The model under review builds one solid part; all positions refer to its coordinate system, in mm. A direction names the side the tool comes from. Coordinates: 2 decimals unless noted, no trailing zeros. Write each loop counter-clockwise with the first axis right and the second up, starting at its lowest first coordinate (ties: lowest second). Pieces come first, ordered by that corner, then holes. Notation, with made-up numbers: M 67,-27.5 L 102,-27.5 A32 cw 102,1.5 Z; hole C -4.75,-16.75 d5. An arc over 180 degrees is marked long. Answer as a JSON object with one key per item and string values.
Autodesk Inventor part; units mm, degrees
ref_plane "YZ Plane" through (0, 0, 0) normal (1, 0, 0) x (0, 1, 0)
ref_plane "XZ Plane" through (0, 0, 0) normal (0, 1, 0) x (-1, 0, 0)
ref_plane "XY Plane" through (0, 0, 0) normal (0, 0, 1) x (1, 0, 0)
sketch "Sketch1" plane through (0, 0, 0) normal (0, 0, 1) x (1, 0, 0)
  line L0 (0, 0) -> (12.7, 0)
  line L1 (12.7, 0) -> (12.7, 25.4)
  line L2 (12.7, 25.4) -> (0, 25.4)
  line L3 (0, 25.4) -> (0, 0)
  line L4 (1.27, 24.13) -> (11.43, 24.13)
  line L5 (11.43, 24.13) -> (11.43, 1.27)
  line L6 (11.43, 1.27) -> (1.27, 1.27)
  line L7 (1.27, 1.27) -> (1.27, 24.13)
  dimension "d0" = 25.4
  dimension "d1" = 12.7
  dimension "d2" = 1.27
extrude "Extrusion1" add sketch "Sketch1" along normal blind 203.2
sketch "Sketch2" plane through (12.7, 0, 0) normal (1, 0, 0) x (0, 0, -1)
  line L0 (-168.1044, 12.7) -> (-15.152, 12.7) construction
  line L1 (0, 0) -> (-203.2, 0) construction
  line L2 (-203.2, 0) -> (-203.2, 25.4)
  line L3 (0, 0) -> (0, 25.4)
  point P0 (-177.8, 12.7)
  point P1 (-25.4, 12.7)
  dimension "d5" = 12.7
  dimension "d6" = 25.4
  dimension "d7" = 25.4
hole "Hole1" at (12.7, 12.7, 177.8) at (12.7, 12.7, 25.4) direction (-1, 0, 0) diameter 3.2639 end through all
sketch "Sketch3" plane through (12.7, 0, 0) normal (1, 0, 0) x (0, 0, -1)
  circle A0 centre (-177.8, 12.7) radius 1.632
  circle A1 centre (-25.4, 12.7) radius 1.632
  line L0 (-214.4228, 12.7) -> (16.7128, 12.7) construction
  point P0 (0, 0)
  point P1 (-139.7, 12.7)
  point P2 (-63.5, 12.7)
  dimension "d18" = 38.1
  dimension "d19" = 38.1
hole "Hole2" at (12.7, 12.7, 139.7) at (12.7, 12.7, 63.5) direction (-1, 0, 0) diameter 6.5278 end through all
sketch "Sketch4" plane through (0, 25.4, 0) normal (0, 1, 0) x (1, 0, 0)
  line L0 (6.35, 23.2485) -> (6.35, -226.9955) construction
  line L1 (12.7, 0) -> (12.7, -203.2) construction
  line L2 (12.7, 0) -> (0, 0)
  line L3 (0, 0) -> (0, -203.2)
  line L4 (12.7, -203.2) -> (0, -203.2)
  line L5 (12.7, 0) -> (12.7, -203.2)
  point P0 (0, 0)
  point P1 (6.35, -31.75)
  point P2 (6.35, -171.45)
  dimension "d27" = 6.35
  dimension "d28" = 31.75
  dimension "d29" = 31.75
hole "Hole3" at (6.35, 25.4, 31.75) at (6.35, 25.4, 171.45) direction (0, -1, 0) diameter 3.2512 end through all
properties part number "000101"
(1) For faces 1 (the face through (6, 24.13, 100)), 2 (the face through (12.06, 12.63, 179.43)), list the 3-axis set-ups (+Z, -Z, +X, -X, +Y, -Y) from which the entire face can be reached by the end or side of a thin tool; tool diameter is ignored.
Results list:
{"face 1": "+Z, -Z", "face 2": "+X, -X"}
(2) Add section B-B on y = 17.75. Give the boundary of the cut face in (x, z).
Results list:
{"outline": "M 0,0 L 1.27,0 L 1.27,203.2 L 0,203.2 Z; M 11.43,0 L 12.7,0 L 12.7,203.2 L 11.43,203.2 Z"}
(3) For pin 1 Ø4 at (y, z) = (12.7, 139.7) entering from +X, flat-tipped, find the tip position at first contact; note if it passes through.
Results list:
{"pin 1": "through"}
(4) Add section C-C on z = 139.7. Give the boundary of the cut face in (x, y), and give its area (3 significant figures).
Results list:
{"outline": "M 0,0 L 12.7,0 L 12.7,9.44 L 11.43,9.44 L 11.43,1.27 L 1.27,1.27 L 1.27,9.44 L 0,9.44 Z; M 0,15.96 L 1.27,15.96 L 1.27,24.13 L 11.43,24.13 L 11.43,15.96 L 12.7,15.96 L 12.7,25.4 L 0,25.4 Z", "area": "73.7 mm²"}
(5) Draft analysis for pull direction Z (two halves, no side actions). For faces 3 (the face through (6.279, 24.756, 169.826)), 4 (the face through (6, 0, 100)), 5 (the face through (0.626, 9.948, 137.945)), 6 (the face through (1, 14, 0)), state which applies: released by +Z, released by -Z, zero draft, split by the parting line, or undercut.
Results list:
{"face 3": "undercut", "face 4": "zero draft", "face 5": "undercut", "face 6": "released by -Z"}
(6) Wall thickness on line 1 along Z through (x, y) = (12.3, 12.7); line 2 along Z through (x, y) = (6.35, 0.4); line 3 along Y through (x, z) = (7.25, 37.5): over which ranges is each line inside the solid? List them lowest first. Write a range as from..to.
Results list:
{"line 1": "0..23.77, 27.03..60.24, 66.76..136.44, 142.96..176.17, 179.43..203.2", "line 2": "0..30.12, 33.38..169.82, 173.08..203.2", "line 3": "0..1.27, 24.13..25.4"}
(7) Add section A-A on z = 40.5. Give the boundary of the cut face in (x, y), and give its area (3 significant figures).
Results list:
{"outline": "M 0,0 L 12.7,0 L 12.7,25.4 L 0,25.4 Z; hole M 1.27,1.27 L 11.43,1.27 L 11.43,24.13 L 1.27,24.13 Z", "area": "90.3 mm²"}
